For this review, take the finished solid that the model builds, in its own axes (mm). Face numbers are marked on the shaded views. A direction names the side the tool comes from. Coordinates: 2 decimals unless noted, no trailing zeros. Loops run counter-clockwise (first coordinate to the right, second up) from the corner with the lowest first, then second, coordinate; pieces in that order, holes last. Notation, with made-up numbers: (43.25, -8.5) -> (99.25, -8.5) arc R14 ccw to (99.25, 16.5) -> close; hole circle Ø10 at (37, 63.5). An arc over 180 degrees is marked (long way). Answer in a Markdown table with one row per item.
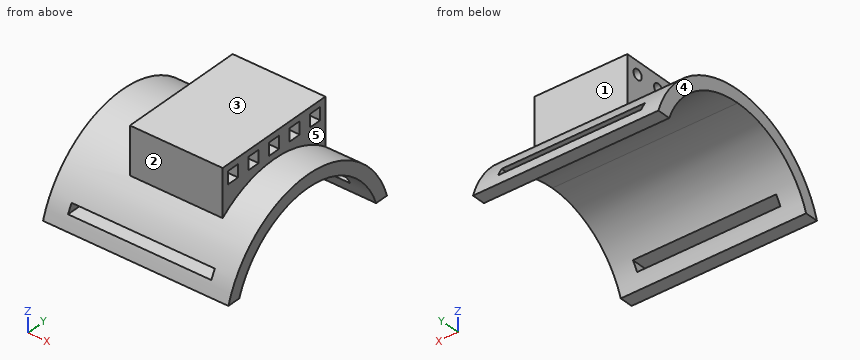
from build123d import *

# Parameters (mm, degrees)
F1_DEPTH      = 55.88
F3_R          = 1.524
F4_DEPTH      = 2.54
F5_W          = 43.18
F5_H          = 2.54
F6_DEPTH      = 54.8232105123
F6_DEPTH_BACK = 25.4
F7_W          = 3.81
F7_H          = 3.81
F8_DEPTH      = 25.4


with BuildPart() as f1:
    # F0 (on Right) → F1 (new body)
    with BuildSketch(Plane.YZ):
        with BuildLine():
            Line((-4.0222105123, 0), (0, 0))
            ThreePointArc((0, 0), (9.897674368, 12.8933223314), (25.4, 17.78))
            ThreePointArc((25.4, 17.78), (40.902325632, 12.8933223314), (50.8, 0))
            Line((50.8, 0), (54.8222105123, 0))
            ThreePointArc((54.8222105123, 0), (25.4, 21.59), (-4.0222105123, 0))
        make_face()
    extrude(amount=F1_DEPTH)

    # F3 (on offset) → F4 (join)
    with BuildSketch(Plane(origin=(17.78, 0, 0), x_dir=(0, -1, 0), z_dir=(-1, 0, 0))):
        with BuildLine():
            ThreePointArc((-44.45, 13.97), (-35.6587389576, 19.614347394), (-25.4, 21.59))
            Line((-25.4, 21.59), (-25.4, 23.876))
            ThreePointArc((-25.4, 23.876), (-26.924, 25.4), (-25.4, 26.924))
            Line((-25.4, 26.924), (-25.4, 29.21))
            Line((-25.4, 29.21), (-44.45, 29.21))
            Line((-44.45, 29.21), (-44.45, 13.97))
        make_face()
        with Locations((-40.64, 25.4)):
            Circle(F3_R, mode=Mode.SUBTRACT)
        with Locations((-33.02, 25.4)):
            Circle(F3_R, mode=Mode.SUBTRACT)
        with BuildLine():
            Line((-25.4, 23.876), (-25.4, 21.59))
            ThreePointArc((-25.4, 21.59), (-15.1412610424, 19.614347394), (-6.35, 13.97))
            Line((-6.35, 13.97), (-6.35, 29.21))
            Line((-6.35, 29.21), (-25.4, 29.21))
            Line((-25.4, 29.21), (-25.4, 26.924))
            ThreePointArc((-25.4, 26.924), (-24.3223692655, 26.4776307345), (-23.876, 25.4))
            ThreePointArc((-23.876, 25.4), (-24.3223692655, 24.3223692655), (-25.4, 23.876))
        make_face()
        with Locations((-17.78, 25.4)):
            Circle(F3_R, mode=Mode.SUBTRACT)
        with Locations((-10.16, 25.4)):
            Circle(F3_R, mode=Mode.SUBTRACT)
    extrude(amount=-F4_DEPTH)

    # F5 (on Front) → F6 (cut, two sides)
    with BuildSketch(Plane.XZ) as f6_sk:
        with Locations((27.94, 5.08)):
            Rectangle(F5_W, F5_H)
    extrude(amount=-F6_DEPTH, mode=Mode.SUBTRACT)
    extrude(f6_sk.sketch, amount=F6_DEPTH_BACK, mode=Mode.SUBTRACT)

    # F7 (on face) → F8 (join)
    with BuildSketch(Plane.YZ.offset(20.32)):
        with BuildLine():
            Line((6.35, 29.21), (6.35, 15.0036746936))
            ThreePointArc((6.35, 15.0036746936), (25.4, 21.59), (44.45, 15.0036746936))
            Line((44.45, 15.0036746936), (44.45, 29.21))
            Line((44.45, 29.21), (6.35, 29.21))
        make_face()
        with Locations((10.16, 25.4)):
            Rectangle(F7_W, F7_H, mode=Mode.SUBTRACT)
        with Locations((17.78, 25.4)):
            Rectangle(F7_W, F7_H, mode=Mode.SUBTRACT)
        with Locations((25.4, 25.4)):
            Rectangle(F7_W, F7_H, mode=Mode.SUBTRACT)
        with Locations((33.02, 25.4)):
            Rectangle(F7_W, F7_H, mode=Mode.SUBTRACT)
        with Locations((40.64, 25.4)):
            Rectangle(F7_W, F7_H, mode=Mode.SUBTRACT)
    extrude(amount=F8_DEPTH)


solid = f1.part
Item 1: Take a section at C-C, the plane y = 33.02. State the section outline as (x, z) points (3 decimals), and give its area (3 significant figures).
Worked answers:
| item | result |
|---|---|
| outline | (0, 16.684) -> (55.88, 16.684) -> (55.88, 20.634) -> (45.72, 20.634) -> (45.72, 23.495) -> (20.32, 23.495) -> (20.32, 23.876) -> (17.78, 23.876) -> (17.78, 20.634) -> (0, 20.634) -> close; (17.78, 26.924) -> (20.32, 26.924) -> (20.32, 27.305) -> (45.72, 27.305) -> (45.72, 29.21) -> (17.78, 29.21) -> close |
| area | 356 mm² |
Item 2: Insertion check: pin 1 (1 mm diameter, centred on x = 48.5, z = 7.5, fed in from -Y); pin 2 (3 mm diameter, centred on x = 29, y = 10.5, fed in from -Z); pin 3 (5 mm diameter, centred on x = 11, y = 28, fed in from -Z); pin 4 (2.5 mm diameter, centred on y = 40.64, z = 25.4, fed in from +X). Each pin has a flat end and moves straight along its axis. Give the tip position at first contact, or say it passes through.
Worked answers:
| item | result |
|---|---|
| pin 1 | y = -0.81 |
| pin 2 | z = 12.24 |
| pin 3 | z = 17.29 |
| pin 4 | through |
Item 3: For L1, parallel to Y at x = 18, z = 18.5; L2, parallel to X at y = 38, z = 24; L3, parallel to Y at x = 49, z = 12, list the stretches that pass through material, from the lowest coordinate up.
Worked answers:
| item | result |
|---|---|
| L1 | 6.35 to 44.45 |
| L2 | 17.78 to 45.72 |
| L3 | 3.05 to 8.69, 42.11 to 47.75 |
Item 4: Take a section at B-B, the plane z = 13. State the section outline as (x, y) points.
Worked answers:
| item | result |
|---|---|
| outline | (0, 4.04) -> (55.88, 4.04) -> (55.88, 10.05) -> (0, 10.05) -> close; (0, 40.75) -> (55.88, 40.75) -> (55.88, 46.76) -> (0, 46.76) -> close |
Item 5: For the marked faces 1, 2, 3, 4 and 5, list the 3-axis set-ups (+Z, -Z, +X, -X, +Y, -Y) from which the entire face can be reached by the end or side of a thin tool; tool diameter is ignored.
Worked answers:
| item | result |
|---|---|
| face 1 | +Z, +X, -X, +Y |
| face 2 | +Z, +X, -X, -Y |
| face 3 | +Z, +X, -X, +Y, -Y |
| face 4 | +Z, -Z, -X, +Y, -Y |
| face 5 | +Z, +X |
Item 6: Take a section at D-D, the plane y = 43.5. State the section outline as (x, z) points.
Worked answers:
| item | result |
|---|---|
| outline | (0, 10.83) -> (55.88, 10.83) -> (55.88, 15.72) -> (45.72, 15.72) -> (45.72, 29.21) -> (17.78, 29.21) -> (17.78, 15.72) -> (0, 15.72) -> close |
Item 7: Take a section at A-A, the plane x = 48.5. State the section outline as (y, z) points.
Worked answers:
| item | result |
|---|---|
| outline | (-4.02, 0) -> (0, 0) arc R27.03 cw to (1.73, 3.81) -> (-2.54, 3.81) arc R30.84 ccw to start; (-1.21, 6.35) -> (3.32, 6.35) arc R27.03 cw to (47.48, 6.35) -> (52.01, 6.35) arc R30.84 ccw to start; (49.07, 3.81) arc R27.03 cw to (50.8, 0) -> (54.82, 0) arc R30.84 ccw to (53.34, 3.81) -> close |
